from build123d import *

# Parameters (mm, degrees)
F1_DEPTH = 55
F3_DEPTH = 5
F4_DEPTH = 5
F5_R     = 10
F6_DEPTH = 10
F7_DEPTH = 15


with BuildPart() as f1:
    # F0 (on Front) → F1 (new body)
    with BuildSketch(Plane.XZ):
        with BuildLine():
            Line((5, 0), (9, 0))
            ThreePointArc((9, 0), (7.9372539332, 4.2426406871), (5, 7.4833147735))
            Line((5, 7.4833147735), (5, 3.0001575886))
            Line((5, 3.0001575886), (5, 0))
        make_face()
        with BuildLine():
            Line((5, 3.0001575886), (5, 7.4833147735))
            ThreePointArc((5, 7.4833147735), (0, 9), (-5, 7.4833147735))
            Line((-5, 7.4833147735), (-5, 3.0001575886))
            ThreePointArc((-5, 3.0001575886), (-4.4142135624, 4.414371151), (-3, 5.0001575886))
            Line((-3, 5.0001575886), (3, 5.0001575886))
            ThreePointArc((3, 5.0001575886), (4.4142135624, 4.414371151), (5, 3.0001575886))
        make_face()
        with BuildLine():
            Line((-5, 3.0001575886), (-5, 7.4833147735))
            ThreePointArc((-5, 7.4833147735), (-7.9372539332, 4.2426406871), (-9, 0))
            Line((-9, 0), (-5, 0))
            Line((-5, 0), (-5, 3.0001575886))
        make_face()
    extrude(amount=F1_DEPTH)

    # F2 (on face) → F3 (join)
    with BuildSketch(Plane.XZ.offset(55)):
        with BuildLine():
            Line((-5, 0), (-5, 3.0001575886))
            Line((-5, 3.0001575886), (-5, 7.4833147735))
            ThreePointArc((-5, 7.4833147735), (-7.9372539332, 4.2426406871), (-9, 0))
            Line((-9, 0), (-5, 0))
        make_face()
        with BuildLine():
            Line((-5, 7.4833147735), (-5, 3.0001575886))
            ThreePointArc((-5, 3.0001575886), (-4.4142135624, 4.414371151), (-3, 5.0001575886))
            Line((-3, 5.0001575886), (3, 5.0001575886))
            ThreePointArc((3, 5.0001575886), (4.4142135624, 4.414371151), (5, 3.0001575886))
            Line((5, 3.0001575886), (5, 7.4833147735))
            ThreePointArc((5, 7.4833147735), (0, 9), (-5, 7.4833147735))
        make_face()
        with BuildLine():
            Line((-5, 9.7981165597), (-5, 7.4833147735))
            ThreePointArc((-5, 7.4833147735), (0, 9), (5, 7.4833147735))
            Line((5, 7.4833147735), (5, 9.7981165597))
            ThreePointArc((5, 9.7981165597), (0, 11.0001403681), (-5, 9.7981165597))
        make_face()
        with BuildLine():
            Line((5, 7.4833147735), (5, 3.0001575886))
            Line((5, 3.0001575886), (5, 0))
            Line((5, 0), (9, 0))
            ThreePointArc((9, 0), (7.9372539332, 4.2426406871), (5, 7.4833147735))
        make_face()
    extrude(amount=F3_DEPTH)



with BuildPart() as f4:
    # F0 (on Front) → F4 (new body)
    with BuildSketch(Plane.XZ):
        with BuildLine():
            Line((-10, -20.2321839634), (10, -20.2321839634))
            ThreePointArc((10, -20.2321839634), (13.5355339059, -18.7677178693), (15, -15.2321839634))
            Line((15, -15.2321839634), (15, 15.2321839634))
            ThreePointArc((15, 15.2321839634), (13.5355339059, 18.7677178693), (10, 20.2321839634))
            Line((10, 20.2321839634), (-10, 20.2321839634))
            ThreePointArc((-10, 20.2321839634), (-13.5355339059, 18.7677178693), (-15, 15.2321839634))
            Line((-15, 15.2321839634), (-15, -15.2321839634))
            ThreePointArc((-15, -15.2321839634), (-13.5355339059, -18.7677178693), (-10, -20.2321839634))
        make_face()
        with BuildLine():
            ThreePointArc((5, 7.4833147735), (7.9372539332, 4.2426406871), (9, 0))
            Line((9, 0), (5, 0))
            Line((5, 0), (5, -3.0001575886))
            ThreePointArc((5, -3.0001575886), (4.4142135624, -4.414371151), (3, -5.0001575886))
            Line((3, -5.0001575886), (-3, -5.0001575886))
            ThreePointArc((-3, -5.0001575886), (-4.4142135624, -4.414371151), (-5, -3.0001575886))
            Line((-5, -3.0001575886), (-5, 0))
            Line((-5, 0), (-9, 0))
            ThreePointArc((-9, 0), (-7.9372539332, 4.2426406871), (-5, 7.4833147735))
            Line((-5, 7.4833147735), (-5, 10.3561575886))
            ThreePointArc((-5, 10.3561575886), (0, 11.5), (5, 10.3561575886))
            Line((5, 10.3561575886), (5, 7.4833147735))
        make_face(mode=Mode.SUBTRACT)
        with BuildLine():
            Line((5, 0), (9, 0))
            ThreePointArc((9, 0), (7.9372539332, 4.2426406871), (5, 7.4833147735))
            Line((5, 7.4833147735), (5, 3.0001575886))
            Line((5, 3.0001575886), (5, 0))
        make_face()
        with BuildLine():
            Line((5, 3.0001575886), (5, 7.4833147735))
            ThreePointArc((5, 7.4833147735), (0, 9), (-5, 7.4833147735))
            Line((-5, 7.4833147735), (-5, 3.0001575886))
            ThreePointArc((-5, 3.0001575886), (-4.4142135624, 4.414371151), (-3, 5.0001575886))
            Line((-3, 5.0001575886), (3, 5.0001575886))
            ThreePointArc((3, 5.0001575886), (4.4142135624, 4.414371151), (5, 3.0001575886))
        make_face()
        with BuildLine():
            Line((-5, 3.0001575886), (-5, 7.4833147735))
            ThreePointArc((-5, 7.4833147735), (-7.9372539332, 4.2426406871), (-9, 0))
            Line((-9, 0), (-5, 0))
            Line((-5, 0), (-5, 3.0001575886))
        make_face()
        with BuildLine():
            ThreePointArc((-5, 7.4833147735), (0, 9), (5, 7.4833147735))
            Line((5, 7.4833147735), (5, 10.3561575886))
            ThreePointArc((5, 10.3561575886), (0, 11.5), (-5, 10.3561575886))
            Line((-5, 10.3561575886), (-5, 7.4833147735))
        make_face()
    extrude(amount=-F4_DEPTH)

    # F5 (on face) → F6 (join)
    with BuildSketch(Plane(origin=(0, 5, 0), x_dir=(-1, 0, 0), z_dir=(0, 1, 0))):
        with BuildLine():
            ThreePointArc((-15, 3.9e-09), (-1.9e-09, -15), (15, 0))
            ThreePointArc((15, 0), (1.9e-09, 15), (-15, 3.9e-09))
        make_face()
        Circle(F5_R, mode=Mode.SUBTRACT)
    extrude(amount=F6_DEPTH)


with BuildPart() as f1_1:
    add(f1.part)

    add(f4.part)  # F7 merges F4
    # F0 (on Front) → F7 (join)
    with BuildSketch(Plane.XZ):
        with BuildLine():
            ThreePointArc((-5, 7.4833147735), (0, 9), (5, 7.4833147735))
            Line((5, 7.4833147735), (5, 10.3561575886))
            ThreePointArc((5, 10.3561575886), (0, 11.5), (-5, 10.3561575886))
            Line((-5, 10.3561575886), (-5, 7.4833147735))
        make_face()
    extrude(amount=F7_DEPTH)


solid = f1_1.part
Can you work these out from the model? Positions are in its coordinate system, mm. A direction names the side the tool comes from. Coordinates: 2 decimals unless noted, no trailing zeros. Write each loop counter-clockwise with the first axis right and the second up, starting at its lowest first coordinate (ties: lowest second). Pieces come first, ordered by that corner, then holes. Notation, with made-up numbers: (-1.75, 63) - (33.25, 63) arc R31 cw to (33.25, 98) - close; hole circle Ø11 at (8.25, 20). An arc over 180 degrees is marked (long way). Return JSON: item names as keys, results as strings. Group by question number.
Item 1: I'm going to push flat-ended pins straight in: pin 1 Ø1.2 at (x, y) = (7.5, -22.5) entering from -Z; pin 2 Ø2.5 at (y, z) = (-57, 9) entering from -X; pin 3 Ø8 at (y, z) = (-30.5, 0.5) entering from +X. Where does each tip first touch, or does it pass through?
Item 2: If we section it at B-B (y = -11): Write out the boundary of the cut face in (x, z).
Item 3: Which directions (+Z, -Z, +X, -X, +Y, -Y) give clear straight access to the entire face, cutting with the end or side of a thin tool? Please do faces 1 (the face through (0, 5, -17)), 2 (the face through (4, 5, 5)), 3 (the face through (5, -28, 1)).
Item 4: If we section it at C-C (z = 6.5): Write out the boundary of the cut face in (x, y), then the cut area to 3 significant figures.
Item 5: If we section it at A-A (x = 0): Write out the boundary of the cut face in (y, z).
Item 6: We'd pull the mould along Z, two halves only. Please class faces 4 (the face through (0.1, -7.4, 11.5)), 5 (the face through (2.17, 9.93, -9.76)), 6 (the face through (-3, 15, -10)): pulls with the +Z half, pulls with the -Z half, needs draft (parallel to the pull), parting line crosses it, or undercut.
Item 7: Please list where these lines run through material, in increasing order: probe 1 along Y at (x, z) = (10.75, 7); probe 2 along Y at (x, z) = (-9.5, 16.5); probe 3 along Z at (x, y) = (0, 9.5).
Item 8: If we section it at D-D (x = -6.25): Write out the boundary of the cut face in (y, z).
Return value:
{
 "1": {"pin 1": "stops at z = 0", "pin 2": "stops at x = -5", "pin 3": "stops at x = 9"},
 "2": {"outline": "(-9, 0) - (-5, 0) - (-5, 3) arc R2 cw to (-3, 5) - (3, 5) arc R2 cw to (5, 3) - (5, 0) - (9, 0) arc R9 ccw to (5, 7.48) - (5, 10.36) arc R11.5 ccw to (-5, 10.36) - (-5, 7.48) arc R9 ccw to start"},
 "3": {"face 1": "-Z, +Y", "face 2": "+Y", "face 3": "+Y, -Y"},
 "4": {"outline": "(-15, 0) - (-6.22, 0) - (-6.22, -60) - (6.22, -60) - (6.22, 0) - (15, 0) - (15, 5) - (13.52, 5) - (13.52, 15) - (7.6, 15) - (7.6, 5) - (-7.6, 5) - (-7.6, 15) - (-13.52, 15) - (-13.52, 5) - (-15, 5) - close", "area": "1,020 mm^2"},
 "5": {"outline": "(-60, 5) - (5, 5) - (5, 10) - (15, 10) - (15, 15) - (5, 15) - (5, 20.23) - (0, 20.23) - (0, 11.5) - (-15, 11.5) - (-15, 9) - (-55, 9) - (-55, 11) - (-60, 11) - close; (0, -20.23) - (5, -20.23) - (5, -15) - (15, -15) - (15, -10) - (5, -10) - (5, -5) - (0, -5) - close"},
 "6": {"face 4": "pulls with the +Z half", "face 5": "undercut", "face 6": "needs draft"},
 "7": {"probe 1": "y = 0 to 15", "probe 2": "y = 0 to 5", "probe 3": "z = -15 to -10, 10 to 15"},
 "8": {"outline": "(-60, 0) - (0, 0) - (0, -20.23) - (5, -20.23) - (5, -13.64) - (15, -13.64) - (15, -7.81) - (5, -7.81) - (5, 7.81) - (15, 7.81) - (15, 13.64) - (5, 13.64) - (5, 20.23) - (0, 20.23) - (0, 6.48) - (-60, 6.48) - close"}
}
